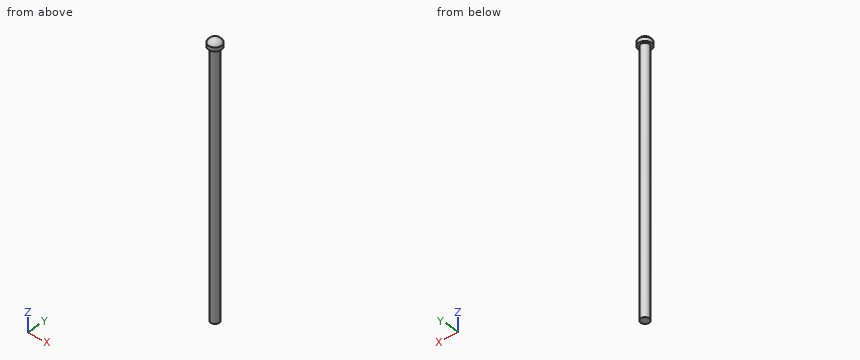
```python
from build123d import *

# Parameters (mm, degrees)
SKETCH2_R           = 3.25
SKETCH8_R           = 5
BOSS_EXTRUDE1_DEPTH = 3
DOME1_FACE_RADIUS   = 5
DOME1_HEIGHT        = 3


with BuildPart() as part:
    # Sweep1: sweep along a path in Sketch7
    with BuildLine(Plane(origin=(0, 0, 0), x_dir=(0, 0, -1), z_dir=(1, 0, 0))) as sweep1_path:
        Line((0, 0), (200, 0))
    # Sketch2 → Sweep1 (sweep)
    with BuildSketch(Plane.XY):
        with Locations((5, 60)):
            Circle(SKETCH2_R)
    sweep(path=sweep1_path.line)

    # Sketch8 → Boss-Extrude1 (add)
    with BuildSketch(Plane.XY):
        with Locations((5, 60)):
            Circle(SKETCH8_R)
    extrude(amount=BOSS_EXTRUDE1_DEPTH)

    # Dome1: a dome of height H over a round flat face of radius A is a cap of a sphere of radius (A * A + H * H) / (2 * H)
    dome1_r = (DOME1_FACE_RADIUS * DOME1_FACE_RADIUS + DOME1_HEIGHT * DOME1_HEIGHT) / (2 * DOME1_HEIGHT)
    dome1_base = Plane((5, 60, 3), z_dir=(0, 0, 1))
    with Locations(dome1_base.offset(DOME1_HEIGHT - dome1_r)):
        dome1_ball = Sphere(dome1_r, mode=Mode.PRIVATE)
    add(split(dome1_ball, bisect_by=dome1_base, keep=Keep.TOP, mode=Mode.PRIVATE))


solid = part.part
```
Verification items for the finished model (mm, model axes). Give positions to 0.01 mm unless a question says otherwise; leave off trailing zeros. Order: outer loops, then holes, each group sorted by start corner. A loop starts at its lowest first (then second) coordinate and runs counter-clockwise, first axis right, second up. Notation, with made-up numbers: (-19, -33) -> (-8, -33) arc R10 cw to (-8, -22) -> close; hole circle Ø3 at (18.25, 69.25). An arc over 180 degrees is marked (long way). Use a Markdown table: item, result.
1) Material ranges on probe 1 along Y at (x, z) = (5.25, -183); probe 2 along X at (y, z) = (60.25, -3); probe 3 along Y at (x, z) = (6.75, -10), recorded low to high.
Results:
| item | result |
|---|---|
| probe 1 | 56.76 to 63.24 |
| probe 2 | 1.76 to 8.24 |
| probe 3 | 57.26 to 62.74 |
2) Depth check by flat-ended pin: pin 1 Ø1.5 at (x, y) = (5.5, 61) entering from +Z; pin 2 Ø5 at (x, y) = (1.5, 58) entering from +Z; pin 3 Ø5 at (y, z) = (61, -146) entering from +X. Enter the tip coordinate at first touch or a pass-through.
Results:
| item | result |
|---|---|
| pin 1 | z = 5.99 |
| pin 2 | z = 5.79 |
| pin 3 | x = 8.25 |
3) Section check C-C, the plane z = -120. Record the boundary of the cut face in (x, y).
Results:
| item | result |
|---|---|
| outline | circle Ø6.5 at (5, 60) |
4) Section check B-B, the plane y = 60. Record the boundary of the cut face in (x, z).
Results:
| item | result |
|---|---|
| outline | (0, 0) -> (1.75, 0) -> (1.75, -200) -> (8.25, -200) -> (8.25, 0) -> (10, 0) -> (10, 3) arc R5.67 ccw to (0, 3) -> close |
5) Section check A-A, the plane x = 5. Record the boundary of the cut face in (y, z), then the cut area to 3 significant figures.
Results:
| item | result |
|---|---|
| outline | (55, 0) -> (56.75, 0) -> (56.75, -200) -> (63.25, -200) -> (63.25, 0) -> (65, 0) -> (65, 3) arc R5.67 ccw to (55, 3) -> close |
| area | 1,350 mm² |
